Geometry: see drawing. Coordinates: mm, zero at the bounding-box minimum. Coordinates: 2 decimals unless noted, no trailing zeros. Loops run counter-clockwise (first coordinate to the right, second up) from the corner with the lowest first, then second, coordinate; pieces in that order, holes last.
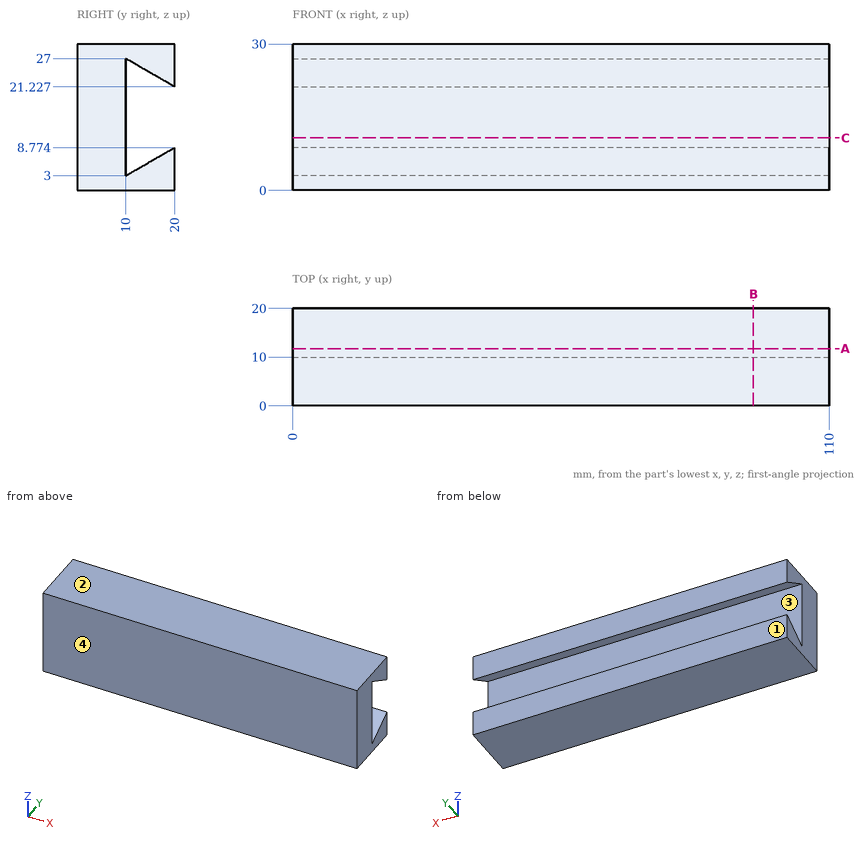
Item 1: Section query C-C (z = 10.75). Output: boundary loops of the cut face in (x, y), then the cut area to 3 significant figures.
Result:
outline: (0, 0) - (110, 0) - (110, 10) - (0, 10) - close
area: 1,100 mm2
Item 2: Section query A-A (y = 11.75). Output: boundary loops of the cut face in (x, z).
Result:
outline: (0, 0) - (110, 0) - (110, 4.01) - (0, 4.01) - close; (0, 25.99) - (110, 25.99) - (110, 30) - (0, 30) - close
Item 3: Mould query, pull axis Y, two halves, no side actions, for the marked faces 1, 2, 3 and 4. Classes: +Y half, -Y half, draft (parallel to the pull), parting line (faces both ways), or undercut.
Result:
face 1: +Y half
face 2: draft
face 3: undercut
face 4: -Y half
Item 4: Line query: L1, parallel to Y at x = 81, z = 16; L2, parallel to Y at x = 37, z = 22.75 (1 decimal); L3, parallel to Y at x = 44.5, z = 6.25 (1 decimal). Output: solid intervals per line, ascending.
Result:
L1: y = 0 to 10
L2: y = 0 to 10, 17.4 to 20
L3: y = 0 to 10, 15.6 to 20
Item 5: Section query B-B (x = 94.5). Output: boundary loops of the cut face in (y, z), then the cut area to 3 significant figures.
Result:
outline: (0, 0) - (20, 0) - (20, 8.77) - (10, 3) - (10, 27) - (20, 21.23) - (20, 30) - (0, 30) - close
area: 418 mm2
